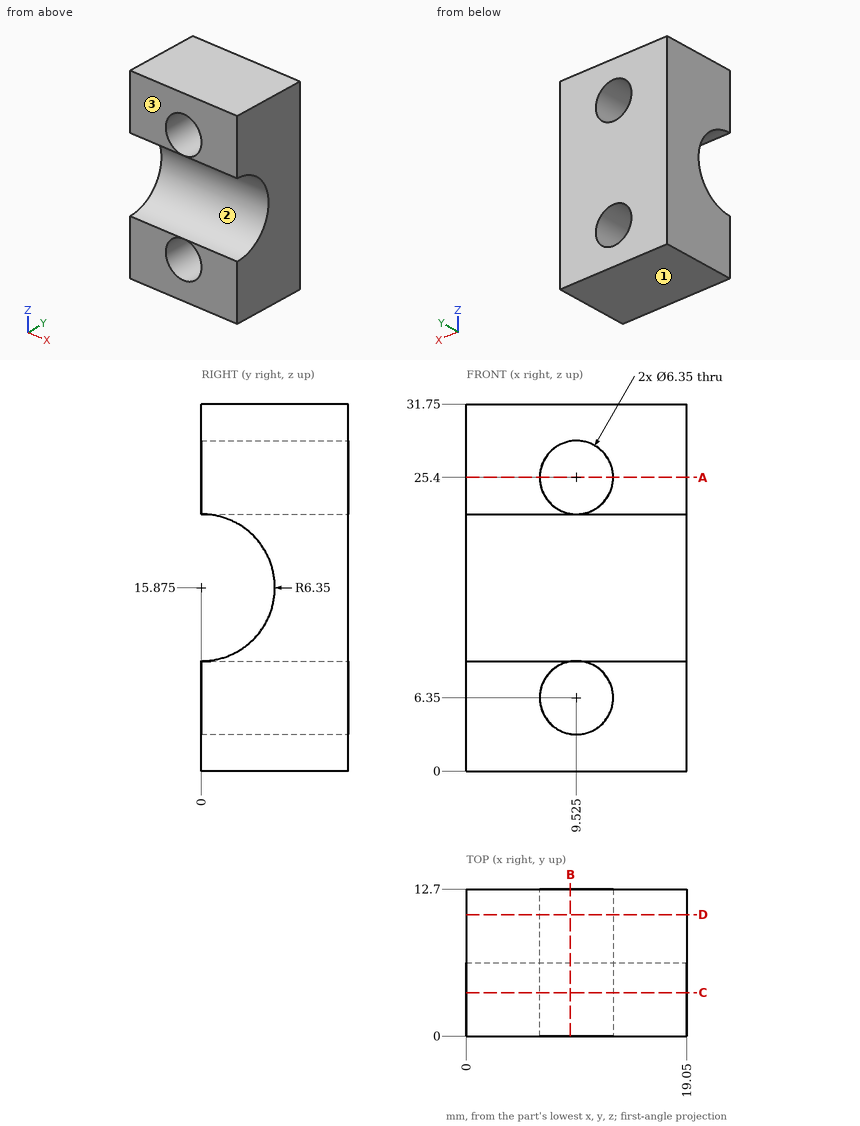
Check sheet for the drawn part. Datum: minimum x, y, z corner. Units: mm. Give positions to 0.01 mm unless a question says otherwise; leave off trailing zeros. Order: outer loops, then holes, each group sorted by start corner. A loop starts at its lowest first (then second) coordinate and runs counter-clockwise, first axis right, second up. Notation, with made-up numbers: (46, 62) -> (84, 62) arc R10 cw to (84, 72) -> close; hole circle Ø6 at (3.5, -22.75). An arc over 180 degrees is marked (long way). One line per item, written item: value.
(1) Sectioned sample at C-C on y = 3.75. Record the cut outline in (x, z) (3 decimals).
Final values:
outline: (0, 0) -> (19.05, 0) -> (19.05, 10.751) -> (0, 10.751) -> close; (0, 20.999) -> (19.05, 20.999) -> (19.05, 31.75) -> (0, 31.75) -> close; hole circle Ø6.35 at (9.525, 6.35); hole circle Ø6.35 at (9.525, 25.4)
(2) Scan lines: line 1 along Z through (x, y) = (9.5, 11.5); line 2 along X through (y, z) = (9, 6.35); line 3 along Z through (x, y) = (10, 9.75). Record each from-to range of solid material in increasing order. Write a range as [from, to].
Final values:
line 1: [0, 3.18], [9.52, 22.23], [28.57, 31.75]
line 2: [0, 6.35], [12.7, 19.05]
line 3: [0, 3.21], [9.49, 22.26], [28.54, 31.75]
(3) Sectioned sample at D-D on y = 10.5. Record the cut outline in (x, z) (3 decimals).
Final values:
outline: (0, 0) -> (19.05, 0) -> (19.05, 31.75) -> (0, 31.75) -> close; hole circle Ø6.35 at (9.525, 6.35); hole circle Ø6.35 at (9.525, 25.4)
(4) Sectioned sample at B-B on x = 9. Record the cut outline in (y, z) (3 decimals).
Final values:
outline: (0, 0) -> (12.7, 0) -> (12.7, 3.219) -> (0, 3.219) -> close; (0, 9.481) -> (12.7, 9.481) -> (12.7, 22.269) -> (0, 22.269) -> (0, 22.225) arc R6.35 cw to (0, 9.525) -> close; (0, 28.531) -> (12.7, 28.531) -> (12.7, 31.75) -> (0, 31.75) -> close
(5) Sectioned sample at A-A on z = 25.4. Record the cut outline in (x, y), then the cut area to 3 significant figures.
Final values:
outline: (0, 0) -> (6.35, 0) -> (6.35, 12.7) -> (0, 12.7) -> close; (12.7, 0) -> (19.05, 0) -> (19.05, 12.7) -> (12.7, 12.7) -> close
area: 161 mm^2
(6) Draft check along Z on the marked faces 1, 2 and 3. Enter one of: pulls with the +Z half, pulls with the -Z half, needs draft (parallel to the pull), parting line crosses it, or undercut.
Final values:
face 1: pulls with the -Z half
face 2: undercut
face 3: needs draft
